from build123d import *

# Parameters (mm, degrees)
SKETCH_1_W          = 23
SKETCH_1_H          = 30
EXTRUDE_2_DEPTH     = 3
EXTRUDE_3_DEPTH     = 18
EXTRUDE_3_2_DEPTH   = 18
EXTRUDE_4_DEPTH     = 23
SKETCH_3_R          = 1.55
CUT_EXTRUDE_2_DEPTH = 35.6
CUT_EXTRUDE_5_DEPTH = 31
SKETCH_9_R          = 1.3
SKETCH_9_R_2        = 3
SKETCH_9_R_3        = 1.55
CUT_EXTRUDE_6_DEPTH = 24
SKETCH_10_R         = 3
CUT_EXTRUDE_7_DEPTH = 2
SKETCH_11_R         = 3
CUT_EXTRUDE_8_DEPTH = 2


with BuildPart() as part:
    # Sketch 1 → Extrude 2 (new body)
    with BuildSketch(Plane(origin=(0, 0, 0), x_dir=(1, 0, 0), z_dir=(0, 1, 0))):
        Rectangle(SKETCH_1_W, SKETCH_1_H)
    extrude(amount=EXTRUDE_2_DEPTH)



with BuildPart() as body_2:
    # Sketch 1_4 → Extrude 3 (new body)
    with BuildSketch(Plane(origin=(0, 0, 0), x_dir=(1, 0, 0), z_dir=(0, 1, 0))):
        Polygon((11.5, -15), (11.5, -11.5), (0, -11.5), (-8.5, -11.5), (-11.5, -11.5), (-11.5, -15), align=None)
    extrude(amount=EXTRUDE_3_DEPTH)


with BuildPart() as body_3:
    # Sketch 1_4 → Extrude 3 2 (new body)
    with BuildSketch(Plane(origin=(0, 0, 0), x_dir=(1, 0, 0), z_dir=(0, 1, 0))):
        Polygon((-11.5, 11.5), (0, 11.5), (11.5, 11.5), (11.5, 15), (-11.5, 15), align=None)
    extrude(amount=EXTRUDE_3_2_DEPTH)


with BuildPart() as part_1:
    add(part.part)

    add(body_2.part)  # Extrude 4 merges body 2

    add(body_3.part)  # Extrude 4 merges body 3
    # Sketch 1_5 → Extrude 4 (add)
    with BuildSketch(Plane(origin=(0, 0, 0), x_dir=(1, 0, 0), z_dir=(0, 1, 0))):
        Polygon((-11.5, 0), (-11.5, 11.5), (-11.5, 15), (-15, 15), (-15, -15), (-11.5, -15), (-11.5, -11.5), align=None)
        Polygon((11.5, 15), (11.5, 11.5), (11.5, 0), (11.5, -11.5), (11.5, -15), (15, -15), (15, 15), align=None)
        Polygon((11.5, -15), (11.5, -11.5), (0, -11.5), (-8.5, -11.5), (-11.5, -11.5), (-11.5, -15), align=None)
        Polygon((-11.5, 11.5), (0, 11.5), (11.5, 11.5), (11.5, 15), (-11.5, 15), align=None)
    extrude(amount=EXTRUDE_4_DEPTH)

    # Sketch 3 → Cut-Extrude 2 (cut, through all)
    with BuildSketch(Plane(origin=(0, 0, -19.6), x_dir=(-1, 0, 0), z_dir=(0, 0, -1))):
        with Locations((0, 10)):
            Circle(SKETCH_3_R)
        with Locations((-7.5, 16)):
            Circle(SKETCH_3_R)
        with Locations((7.5, 16)):
            Circle(SKETCH_3_R)
    extrude(amount=-CUT_EXTRUDE_2_DEPTH, mode=Mode.SUBTRACT)

    # Sketch 8 → Cut-Extrude 5 (cut, through all)
    with BuildSketch(Plane.ZY.offset(15)):
        Polygon((10, 3), (10, 10), (10, 13), (-10, 13), (-10, 3), (0, 3), align=None)
    extrude(amount=-CUT_EXTRUDE_5_DEPTH, mode=Mode.SUBTRACT)

    # Sketch 9 → Cut-Extrude 6 (cut, through all)
    with BuildSketch(Plane.XZ):
        with Locations((-4.949747468, -4.949747468)):
            Circle(SKETCH_9_R)
        with Locations((4.949747468, -4.949747468)):
            Circle(SKETCH_9_R)
        with Locations((4.949747468, 4.949747468)):
            Circle(SKETCH_9_R)
        with Locations((-4.949747468, 4.949747468)):
            Circle(SKETCH_9_R)
        Circle(SKETCH_9_R_2)
        with Locations((7, 0)):
            Circle(SKETCH_9_R_3)
        with Locations((0, 7)):
            Circle(SKETCH_9_R_3)
        with Locations((0, -7)):
            Circle(SKETCH_9_R_3)
        with Locations((-7, 0)):
            Circle(SKETCH_9_R_3)
    extrude(amount=-CUT_EXTRUDE_6_DEPTH, mode=Mode.SUBTRACT)

    # Sketch 10 → Cut-Extrude 7 (cut)
    with BuildSketch(Plane(origin=(0, 0, -15), x_dir=(-1, 0, 0), z_dir=(0, 0, -1))):
        with Locations((7.5, 16)):
            Circle(SKETCH_10_R)
        with Locations((0, 10)):
            Circle(SKETCH_10_R)
        with Locations((-7.5, 16)):
            Circle(SKETCH_10_R)
    extrude(amount=-CUT_EXTRUDE_7_DEPTH, mode=Mode.SUBTRACT)

    # Sketch 11 → Cut-Extrude 8 (cut)
    with BuildSketch(Plane.XY.offset(15)):
        with Locations((-7.5, 16)):
            Circle(SKETCH_11_R)
        with Locations((0, 10)):
            Circle(SKETCH_11_R)
        with Locations((7.5, 16)):
            Circle(SKETCH_11_R)
    extrude(amount=-CUT_EXTRUDE_8_DEPTH, mode=Mode.SUBTRACT)


solid = part_1.part
Work out the finished part from the listing and answer in its coordinate system (mm). A direction names the side the tool comes from. Give positions to 0.01 mm unless a question says otherwise; leave off trailing zeros. Loops run counter-clockwise (first coordinate to the right, second up) from the corner with the lowest first, then second, coordinate; pieces in that order, holes last. Notation, with made-up numbers: (28.25, -8) - (55.25, -8) arc R23 ccw to (55.25, 23) - close; hole circle Ø11 at (-25.75, 61). An arc over 180 degrees is marked (long way). Answer in a Markdown table with one row per item.
(1) Consider L1, parallel to Z at x = 6, y = 12.75; L2, parallel to Z at x = 2.25, y = 8.75. Determine where each line is inside the solid, lowest interval first. Write a range as [from, to].
Results list:
| item | result |
|---|---|
| L1 | z = [-15, -11.5], [11.5, 15] |
| L2 | z = [-13, -11.5], [11.5, 13] |
(2) Section C-C (y = 10) is taken. State how many separate pieces and enclosed holes the cut face has, and give its area (3 significant figures).
Results list:
| item | result |
|---|---|
| separate pieces | 4 |
| enclosed holes | 0 |
| area | 198 mm² |
(3) Section D-D (y = 21) is taken. Give the vertices of the cut face in (x, z), and give its area (3 significant figures).
Results list:
| item | result |
|---|---|
| outline | (-15, -15) - (15, -15) - (15, 15) - (-15, 15) - close; hole (-11.5, -11.5) - (11.5, -11.5) - (11.5, 11.5) - (-11.5, 11.5) - close |
| area | 371 mm² |
(4) Section B-B (y = 4.75) is taken. Give the vertices of the cut face in (x, z).
Results list:
| item | result |
|---|---|
| outline | (-15, -15) - (15, -15) - (15, -10) - (11.5, -10) - (11.5, -11.5) - (-11.5, -11.5) - (-11.5, -10) - (-15, -10) - close; (-15, 10) - (-11.5, 10) - (-11.5, 11.5) - (11.5, 11.5) - (11.5, 10) - (15, 10) - (15, 15) - (-15, 15) - close |
(5) Flat-ended cylindrical pins translate along their axes: pin 1 Ø5 at (x, y) = (7.5, 16) entering from -Z; pin 2 Ø5 at (x, z) = (0, -7) entering from +Y; pin 3 Ø3.5 at (x, y) = (0, 10) entering from +Z. Find the tip coordinate at first contact, or state that the pin passes through.
Results list:
| item | result |
|---|---|
| pin 1 | stops at z = -13 |
| pin 2 | stops at y = 3 |
| pin 3 | stops at z = 13 |
(6) Section A-A (z = -7) is taken. Give the vertices of the cut face in (x, y), and give its area (3 significant figures).
Results list:
| item | result |
|---|---|
| outline | (-15, 0) - (-1.55, 0) - (-1.55, 3) - (-15, 3) - close; (-15, 13) - (-11.5, 13) - (-11.5, 23) - (-15, 23) - close; (1.55, 0) - (15, 0) - (15, 3) - (1.55, 3) - close; (11.5, 13) - (15, 13) - (15, 23) - (11.5, 23) - close |
| area | 151 mm² |
(7) For a pull along Z with two mould halves and no side action, classify faces 1 (the face through (-13, 13, 0)), 2 (the face through (-9, 15, -13)), 3 (the face through (-6.116, 13.338, 14.014)), 4 (the face through (0, 14, 15)) as pulls with the +Z half, pulls with the -Z half, needs draft (parallel to the pull), parting line crosses it, or undercut.
Results list:
| item | result |
|---|---|
| face 1 | undercut |
| face 2 | pulls with the -Z half |
| face 3 | needs draft |
| face 4 | pulls with the +Z half |
(8) A tool of negligible diameter and unlimited length cuts with its end or side. For faces 5 (the face through (0, 13, -11.5)), 6 (the face through (-13, 8, 10)), 7 (the face through (1.3, 8.7, 13)), from which of +Z, -Z, +X, -X, +Y, -Y can it reach the whole face along a straight path? Write none if from no direction.
Results list:
| item | result |
|---|---|
| face 5 | +Y |
| face 6 | +X, -X |
| face 7 | +Z |
